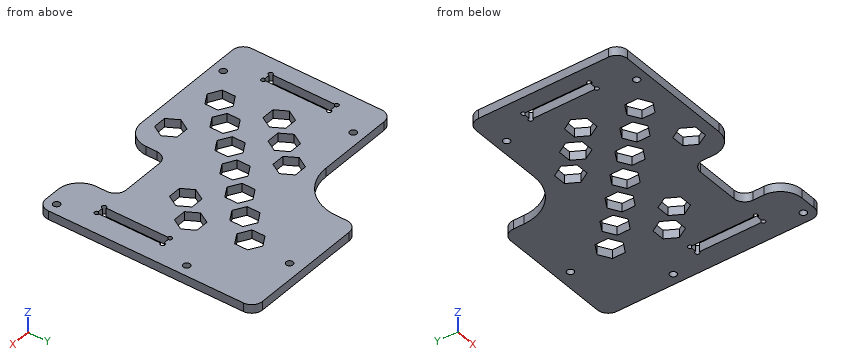
from build123d import *

# Parameters (mm, degrees)
SKETCH_1_W          = 120
SKETCH_1_H          = 70
EXTRUDE_1_DEPTH     = 4
SKETCH_2_W          = 4.4
SKETCH_2_H          = 30.4
CUT_EXTRUDE_1_DEPTH = 139.982013225
SKETCH_3_R          = 1
SKETCH_3_R_2        = 1.575
CUT_EXTRUDE_2_DEPTH = 139.982013225
EXTRUDE_2_DEPTH     = 4
SKETCH_5_R          = 1.575
SKETCH_5_W          = 30
SKETCH_5_H          = 20
CUT_EXTRUDE_3_DEPTH = 141.712472795
FILLET_1_R          = 10
FILLET_2_R          = 5
FILLET_3_R          = 20


with BuildPart() as part:
    # 草图1 → 凸台-拉伸1 (new body)
    with BuildSketch(Plane.XY):
        with Locations((60, -35)):
            Rectangle(SKETCH_1_W, SKETCH_1_H)
    extrude(amount=EXTRUDE_1_DEPTH)

    # 草图2 → 切除-拉伸1 (cut, through all)
    with BuildSketch(Plane.XY.offset(4)):
        with Locations((10, -35)):
            Rectangle(SKETCH_2_W, SKETCH_2_H)
        with Locations((110, -35)):
            Rectangle(SKETCH_2_W, SKETCH_2_H)
    extrude(amount=-CUT_EXTRUDE_1_DEPTH, mode=Mode.SUBTRACT)

    # 草图3 → 切除-拉伸2 (cut, through all)
    with BuildSketch(Plane.XY.offset(4)):
        with Locations((7.8, -19.8)):
            Circle(SKETCH_3_R)
        with Locations((12.2, -19.8)):
            Circle(SKETCH_3_R)
        with Locations((7.8, -50.2)):
            Circle(SKETCH_3_R)
        with Locations((12.2, -50.2)):
            Circle(SKETCH_3_R)
        with Locations((107.8, -19.8)):
            Circle(SKETCH_3_R)
        with Locations((107.8, -50.2)):
            Circle(SKETCH_3_R)
        with Locations((112.2, -50.2)):
            Circle(SKETCH_3_R)
        with Locations((112.2, -19.8)):
            Circle(SKETCH_3_R)
        with Locations((17, -5)):
            Circle(SKETCH_3_R_2)
        with Locations(Location((17, -65, 0), (0, 0, 180))):
            Circle(SKETCH_3_R_2)
        with Locations((117, -5)):
            Circle(SKETCH_3_R_2)
        with Locations(Location((117, -65, 0), (0, 0, 180))):
            Circle(SKETCH_3_R_2)
    extrude(amount=-CUT_EXTRUDE_2_DEPTH, mode=Mode.SUBTRACT)

    # 草图4 → 凸台-拉伸2 (add)
    with BuildSketch(Plane.XY.offset(4)):
        Polygon((60, 0), (60, 30), (122, 30), (122, -70), (120, -70), (120, 0), align=None)
    extrude(amount=-EXTRUDE_2_DEPTH)

    # 草图5 → 切除-拉伸3 (cut, through all)
    with BuildSketch(Plane.XY.offset(4)):
        with Locations((93, 24)):
            Circle(SKETCH_5_R)
        with Locations((84.8, -60)):
            Rectangle(SKETCH_5_W, SKETCH_5_H)
        Polygon((90.8, -2), (95.996152423, 1), (95.996152423, 7), (90.8, 10), (85.603847577, 7), (85.603847577, 1), align=None)
        Polygon((86.096657486, -2.899494937), (80.900505063, 0.100505063), (75.704352641, -2.899494937), (75.704352641, -8.899494937), (80.900505063, -11.899494937), (86.096657486, -8.899494937), align=None)
        Polygon((76.197162549, -12.798989873), (71.001010127, -9.798989873), (65.804857704, -12.798989873), (65.804857704, -18.798989873), (71.001010127, -21.798989873), (76.197162549, -18.798989873), align=None)
        Polygon((66.297667613, -22.69848481), (61.10151519, -19.69848481), (55.905362767, -22.69848481), (55.905362767, -28.69848481), (61.10151519, -31.69848481), (66.297667613, -28.69848481), align=None)
        Polygon((56.398172676, -32.597979746), (51.202020254, -29.597979746), (46.005867831, -32.597979746), (46.005867831, -38.597979746), (51.202020254, -41.597979746), (56.398172676, -38.597979746), align=None)
        Polygon((46.49867774, -42.497474683), (41.302525317, -39.497474683), (36.106372894, -42.497474683), (36.106372894, -48.497474683), (41.302525317, -51.497474683), (46.49867774, -48.497474683), align=None)
        Polygon((36.599182803, -52.39696962), (31.40303038, -49.39696962), (26.206877958, -52.39696962), (26.206877958, -58.39696962), (31.40303038, -61.39696962), (36.599182803, -58.39696962), align=None)
        Polygon((91.143145751, -29.941125497), (88.143145751, -35.13727792), (82.143145751, -35.13727792), (79.143145751, -29.941125497), (82.143145751, -24.744973074), (88.143145751, -24.744973074), align=None)
        Polygon((101.042640687, -20.04163056), (98.042640687, -25.237782983), (92.042640687, -25.237782983), (89.042640687, -20.04163056), (92.042640687, -14.845478138), (98.042640687, -14.845478138), align=None)
        Polygon((61.444660941, -59.639610307), (58.444660941, -64.835762729), (52.444660941, -64.835762729), (49.444660941, -59.639610307), (52.444660941, -54.443457884), (58.444660941, -54.443457884), align=None)
        Polygon((31.05988463, -21.455844123), (34.05988463, -16.2596917), (40.05988463, -16.2596917), (43.05988463, -21.455844123), (40.05988463, -26.651996545), (34.05988463, -26.651996545), align=None)
        Polygon((30.160389693, -36.551491482), (24.160389693, -36.551491482), (21.160389693, -31.355339059), (24.160389693, -26.159186637), (30.160389693, -26.159186637), (33.160389693, -31.355339059), align=None)
        Polygon((43.959379566, -16.752501609), (40.959379566, -11.556349186), (43.959379566, -6.360196763), (49.959379566, -6.360196763), (52.959379566, -11.556349186), (49.959379566, -16.752501609), align=None)
    extrude(amount=-CUT_EXTRUDE_3_DEPTH, mode=Mode.SUBTRACT)

    # 圆角1
    fillet_1_edges = [part.edges().sort_by_distance(p)[0] for p in [
        (69.8, -70, 2),
        (99.8, -70, 2),
    ]]
    fillet(fillet_1_edges, radius=FILLET_1_R)

    # 圆角2
    fillet_2_edges = [part.edges().sort_by_distance(p)[0] for p in [
        (60, 30, 2),
        (122, 30, 2),
        (122, -70, 2),
        (69.8, -50, 2),
        (99.8, -50, 2),
        (0, 0, 2),
        (0, -70, 2),
    ]]
    fillet(fillet_2_edges, radius=FILLET_2_R)

    # 圆角3
    fillet_3_edges = [part.edges().sort_by_distance(p)[0] for p in [
        (60, 0, 2),
    ]]
    fillet(fillet_3_edges, radius=FILLET_3_R)


solid = part.part
Here's how the part is built. I have some questions about the finished solid (model axes, mm). Coordinates: 2 decimals unless noted, no trailing zeros. Loops run counter-clockwise (first coordinate to the right, second up) from the corner with the lowest first, then second, coordinate; pieces in that order, holes last.
1. Imagine slicing it at A-A, the plane x = 17. Please give me the cut outline in (y, z) (3 decimals), and give its area (3 significant figures).
2. Imagine slicing it at B-B, the plane z = 2.1. Count the separate pieces of the cut face and the enclosed holes in it, and give its area (3 significant figures).
3. I need wall thicknesses on L1, parallel to Y at x = 117, z = 2.5 (3 decimals); L2, parallel to X at y = -37, z = 2.25; L3, parallel to Y at x = 27, z = 3.3. Which ranges of each line are inside material? Lowest first, please.
4. For P1, Ø2.5, axis at x = 112.2, y = -19.8, coming from the -Z side; P2, Ø1.9, axis at x = 10, z = 3, coming from the +Y side; P3, Ø1.2, axis at x = 54, z = 1.5, coming from the +Y side, each with a flat end and sliding along its axis, tell me the tip position at first contact or that it passes through.
Taken from the geometry:
1. outline: (-70, 0) - (-66.575, 0) - (-66.575, 4) - (-70, 4) - close; (-63.425, 0) - (-6.575, 0) - (-6.575, 4) - (-63.425, 4) - close; (-3.425, 0) - (0, 0) - (0, 4) - (-3.425, 4) - close
1. area: 255 mm2
2. separate pieces: 1
2. enclosed holes: 20
2. area: 8,290 mm2
3. L1: y = -70 to -66.575, -63.425 to -6.575, -3.425 to 30
3. L2: x = 0 to 7.8, 12.2 to 46.01, 56.4 to 107.8, 112.2 to 122
3. L3: y = -70 to -58.85, -51.94 to -36.55, -26.16 to 0
4. P1: stops at z = 0
4. P2: stops at y = 0
4. P3: stops at y = 6.33
